Geometry check sheet. Reference: drawing and pictorial views, mm from the part's lowest x, y, z. A direction names the side the tool comes from. Round coordinates to 2 decimals unless told otherwise and drop trailing zeros. Order: outer loops, then holes, each group sorted by start corner. A loop starts at its lowest first (then second) coordinate and runs counter-clockwise, first axis right, second up. Notation, with made-up numbers: (85.25, 43.5) -> (121.25, 43.5) arc R14 ccw to (121.25, 67.5) -> close; hole circle Ø9 at (71, -33). An arc over 180 degrees is marked (long way). Return JSON: item names as keys, results as strings. Group by question number.
1) Tool access check on the marked faces 1 and 2. Record the directions out of +Z, -Z, +X, -X, +Y, -Y that give a thin tool (end or side, any length) a straight path to the whole face; none if there is none.
2) Section check B-B on y = 38. Enter the section's corners in (x, z), plus the area to 3 significant figures.
3) Section check C-C on x = 4. State how many separate pieces and enclosed holes the cut face has, plus the area to 3 significant figures.
4) Section check D-D on z = 22.75. Enter the section's corners in (x, y), plus the area to 3 significant figures.
5) Depth check by flat-ended pin: pin 1 (1.5 mm diameter, centred on y = 31, z = 26, fed in from +X); pin 2 (5 mm diameter, centred on y = 12.44, z = 15, fed in from -X); pin 3 (15 mm diameter, centred on x = 27.5, z = 20, fed in from +Y). Enter the tip coordinate at first touch or a pass-through.
6) Section check A-A on z = 15. Enter the section's corners in (x, y).
7) Scan line: L1, parallel to Y at x = 20.5, z = 7.75. Record every from-to range of solid material in increasing order.
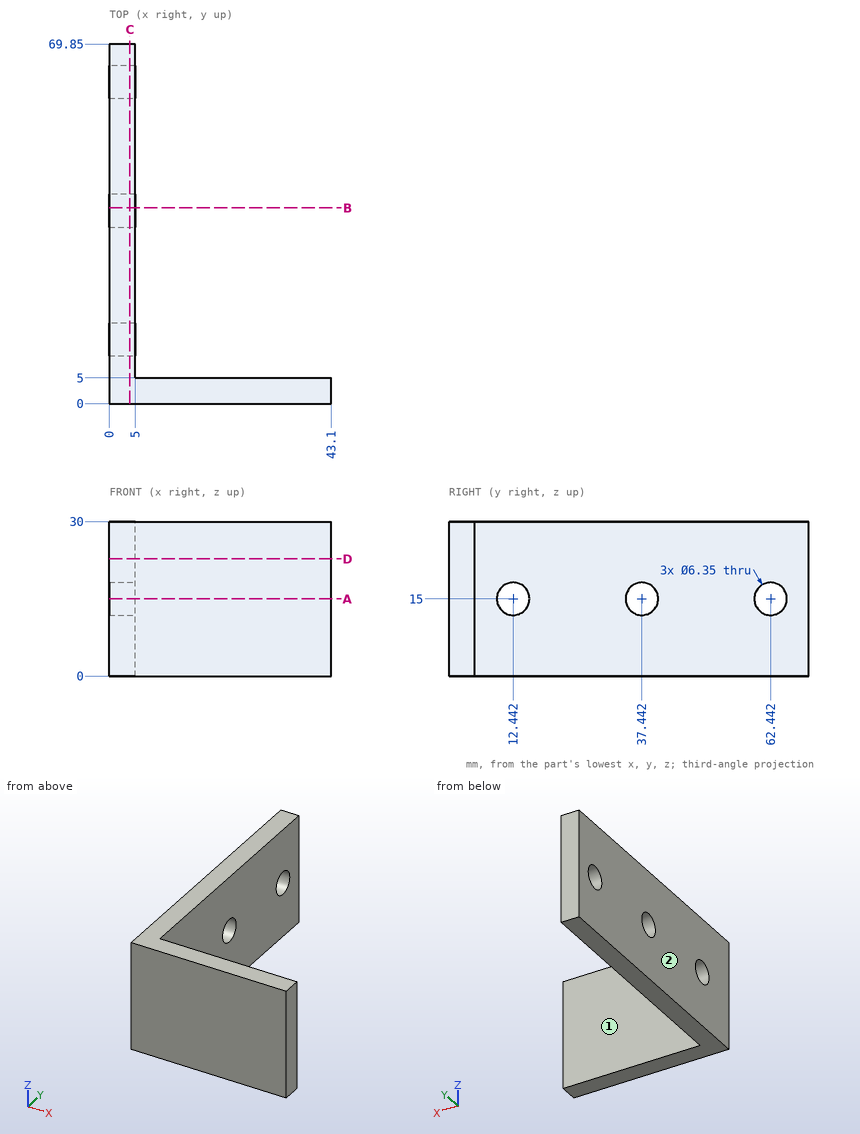
Check result:
{
 "1": {"face 1": "+Z, -Z, +X, +Y", "face 2": "+Z, -Z, -X, +Y, -Y"},
 "2": {"outline": "(0, 0) -> (5, 0) -> (5, 11.87) -> (0, 11.87) -> close; (0, 18.13) -> (5, 18.13) -> (5, 30) -> (0, 30) -> close", "area": "119 mm^2"},
 "3": {"separate pieces": "1", "enclosed holes": "3", "area": "2,000 mm^2"},
 "4": {"outline": "(0, 0) -> (43.1, 0) -> (43.1, 5) -> (5, 5) -> (5, 69.85) -> (0, 69.85) -> close", "area": "540 mm^2"},
 "5": {"pin 1": "x = 5", "pin 2": "through", "pin 3": "y = 5"},
 "6": {"outline": "(0, 0) -> (43.1, 0) -> (43.1, 5) -> (5, 5) -> (5, 9.27) -> (0, 9.27) -> close; (0, 15.62) -> (5, 15.62) -> (5, 34.27) -> (0, 34.27) -> close; (0, 40.62) -> (5, 40.62) -> (5, 59.27) -> (0, 59.27) -> close; (0, 65.62) -> (5, 65.62) -> (5, 69.85) -> (0, 69.85) -> close"},
 "7": {"L1": "0 to 5"}
}
